Geometry check sheet. Reference: the model listing, model coordinates, mm. A direction names the side the tool comes from. Round coordinates to 2 decimals unless told otherwise and drop trailing zeros. Write each loop counter-clockwise with the first axis right and the second up, starting at its lowest first coordinate (ties: lowest second). Pieces come first, ordered by that corner, then holes.
Item 1: Draft check along X on faces 1 (the face through (-1, 1, 9)), 2 (the face through (41.091, 41.293, 6.577)), 3 (the face through (-41.293, 41.091, 6.577)). Enter one of: pulls with the +X half, pulls with the -X half, needs draft (parallel to the pull), parting line crosses it, or undercut.
Item 2: Scan lines: probe 1 along Y at (x, z) = (0, 11.5); probe 2 along Z at (x, y) = (14, -0.5); probe 3 along Y at (x, z) = (-20.5, 9.5). Record each from-to range of solid material in increasing order.
Item 3: Cross-section at C-C (z = 7.5). Enter the section's corners in (x, y).
Item 4: Cross-section at A-A (x = 0). Enter the section's corners in (y, z), then the cut area to 3 significant figures.
Item 5: Access from +Z, -Z, +X, -X, +Y, -Y to the whole of each face (thin tool, end or side, straight path). Record for faces 4 (the face through (-1, 1, 0)), 5 (the face through (-4.88, 37.18, 11.01)).
Item 6: Depth check by flat-ended pin: P1, Ø8, axis at x = -12, y = -10.5, coming from the +Z side. Enter the tip coordinate at first touch or a pass-through.
from build123d import *

# Parameters (mm, degrees)
F0_W     = 90
F0_H     = 90
F1_DEPTH = 13
F2_R     = 37.5
F3_DEPTH = 4
F4_R     = 13
F5_R     = 1


with BuildPart() as f1:
    # F0 (on Top) → F1 (new body)
    with BuildSketch(Plane.XY):
        Rectangle(F0_W, F0_H)
    extrude(amount=F1_DEPTH)

    # F2 (on face) → F3 (cut)
    with BuildSketch(Plane.XY.offset(13)):
        Circle(F2_R)
    extrude(amount=-F3_DEPTH, mode=Mode.SUBTRACT)

    # F4
    f4_edges = [f1.edges().sort_by_distance(p)[0] for p in [
        (45, 45, 6.5),
        (-45, 45, 6.5),
        (-45, -45, 6.5),
        (45, -45, 6.5),
    ]]
    fillet(f4_edges, radius=F4_R)

    # F5
    f5_edges = [f1.edges().sort_by_distance(p)[0] for p in [
        (45, 0, 13),
        (0, 45, 0),
        (37.5, 0, 11),
        (-37.5, 0, 13),
        (-37.5, 0, 9),
    ]]
    fillet(f5_edges, radius=F5_R)


solid = f1.part
Resolved:
1. face 1: undercut
1. face 2: pulls with the +X half
1. face 3: pulls with the -X half
2. probe 1: y = -45 to -37.5, 37.5 to 45
2. probe 2: z = 0 to 9
2. probe 3: y = -45 to -31.24, 31.24 to 45
3. outline: (-45, -32) arc R13 ccw to (-32, -45) - (32, -45) arc R13 ccw to (45, -32) - (45, 32) arc R13 ccw to (32, 45) - (-32, 45) arc R13 ccw to (-45, 32) - close
4. outline: (-45, 1) arc R1 ccw to (-44, 0) - (44, 0) arc R1 ccw to (45, 1) - (45, 12) arc R1 ccw to (44, 13) - (38.5, 13) arc R1 ccw to (37.5, 12) - (37.5, 10) arc R1 cw to (36.5, 9) - (-36.5, 9) arc R1 cw to (-37.5, 10) - (-37.5, 12) arc R1 ccw to (-38.5, 13) - (-44, 13) arc R1 ccw to (-45, 12) - close
4. area: 869 mm2
5. face 4: -Z, +X, -X, +Y, -Y
5. face 5: +Z
6. P1: stops at z = 9
